Part model, mm, in its own coordinate system. A direction names the side the tool comes from. Round coordinates to 2 decimals unless told otherwise and drop trailing zeros. Loops run counter-clockwise (first coordinate to the right, second up) from the corner with the lowest first, then second, coordinate; pieces in that order, holes last. Notation, with made-up numbers: (22.25, 25) -> (71.25, 25) arc R33 ccw to (71.25, 62) -> close; hole circle Ø1 at (0, -40). An arc over 180 degrees is marked (long way). Use a Markdown table: item, result. Add a question column.
Item 1: Flat gauge pins, fed straight in: pin 1 (15 mm diameter, centred on y = -10.5, z = 20.5, fed in from +X); pin 2 (2 mm diameter, centred on x = 2.5, y = -3, fed in from +Z). Where does each tip first touch, or does it go through?
Item 2: Cut at C-C, the plane x = 4. List the corners of the cut face in (y, z), plus the area to 3 significant figures.
Item 3: Probe line 1 (Z direction, x = 17, y = -19.25); line 2 (X direction, y = -19.75, z = 10.25); line 3 (Z direction, x = -8.5, y = -7). List the from-to ranges inside material, lowest first. Write a range as [from, to].
Item 4: Cut at D-D, the plane y = -5.75. List the corners of the cut face in (x, z), plus the area to 3 significant figures.
Item 5: Which spindle directions (+Z, -Z, +X, -X, +Y, -Y) get a long thin tool onto all of the face, cutting with end or side? Do faces 1 (the face through (19, -13, 6.35)), 2 (the face through (7, 0, 4)). Say none if no direction does.
Item 6: Cut at A-A, the plane y = -12.7. List the corners of the cut face in (x, z), plus the area to 3 significant figures.
Item 7: Cut at B-B, the plane z = 23.75. List the corners of the cut face in (x, y).
```python
from build123d import *

# Parameters (mm, degrees)
F0_W     = 38.1
F0_H     = 6.35
F1_DEPTH = 25.4
F3_DEPTH = 12.7


with BuildPart() as f1:
    # F0 (on Front) → F1 (new body)
    with BuildSketch(Plane.XZ):
        with Locations((19.05, 3.175)):
            Rectangle(F0_W, F0_H)
    extrude(amount=F1_DEPTH)

    # F2 (on face) → F3 (join)
    with BuildSketch(Plane(origin=(0, 0, 0), x_dir=(0, -1, 0), z_dir=(-1, 0, 0))):
        with BuildLine():
            Line((0, 12.7), (0, 0))
            Line((0, 0), (25.4, 0))
            Line((25.4, 0), (25.4, 12.7))
            ThreePointArc((25.4, 12.7), (12.7, 25.4), (0, 12.7))
        make_face()
    extrude(amount=F3_DEPTH)


solid = f1.part
```
A:
| question | item | result |
|---|---|---|
| 1 | pin 1 | stops at x = 0 |
| 1 | pin 2 | stops at z = 6.35 |
| 2 | outline | (-25.4, 0) -> (0, 0) -> (0, 6.35) -> (-25.4, 6.35) -> close |
| 2 | area | 161 mm^2 |
| 3 | line 1 | z = [0, 6.35] |
| 3 | line 2 | x = [-12.7, 0] |
| 3 | line 3 | z = [0, 24.05] |
| 4 | outline | (-12.7, 0) -> (38.1, 0) -> (38.1, 6.35) -> (0, 6.35) -> (0, 23.33) -> (-12.7, 23.33) -> close |
| 4 | area | 538 mm^2 |
| 5 | face 1 | +Z, +X, +Y, -Y |
| 5 | face 2 | +Z, -Z, +X, -X, +Y |
| 6 | outline | (-12.7, 0) -> (38.1, 0) -> (38.1, 6.35) -> (0, 6.35) -> (0, 25.4) -> (-12.7, 25.4) -> close |
| 6 | area | 565 mm^2 |
| 7 | outline | (-12.7, -18.96) -> (0, -18.96) -> (0, -6.44) -> (-12.7, -6.44) -> close |
